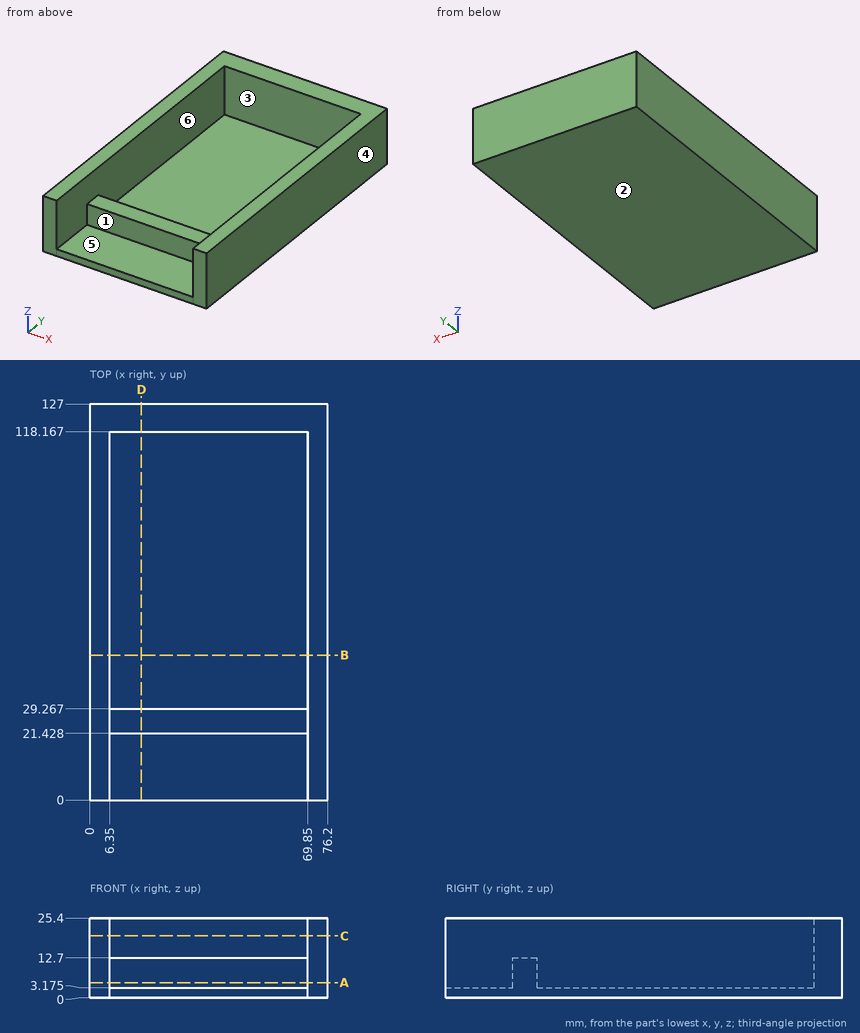
Could you check a few things on this drawing? It's one solid part, dimensions in mm from its lowest x, y, z. A direction names the side the tool comes from. Round coordinates to 2 decimals unless told otherwise and drop trailing zeros. Write each loop counter-clockwise with the first axis right and the second up, starting at its lowest first coordinate (ties: lowest second). Pieces come first, ordered by that corner, then holes.
Q1. If we section it at C-C on z = 19.75: Write out the boundary of the cut face in (x, y), plus the area to 3 significant figures.
Q2. Which directions (+Z, -Z, +X, -X, +Y, -Y) give clear straight access to the entire face, cutting with the end or side of a thin tool? Please do the marked faces 4, 5 and 6.
Q3. If we section it at A-A on z = 4.75: Write out the boundary of the cut face in (x, y).
Q4. Will these pins go through, and if not, where does the flat tip stop? P1, Ø6.5, axis at x = 34, y = 12.5, coming from the +Z side (3 decimals); P2, Ø2, axis at y = 103, z = 11, coming from the -X side; P3, Ø8, axis at x = 59, z = 13, coming from the -Y side; P4, Ø8.5, axis at x = 31, y = 26.5, coming from the +Z side.
Q5. If we mould it in two halves opening along Y, with no side actions, what happens to the marked faces 1, 2 and 3? For each: +Y half, -Y half, draft (parallel to the pull), parting line (faces both ways), or undercut.
Q6. If we section it at B-B on y = 46.5: Write out the boundary of the cut face in (x, z) (3 decimals), plus the area to 3 significant figures.
Q7. Please list where these lines run through material, in increasing order: probe 1 along X at (y, z) = (13, 20); probe 2 along Y at (x, z) = (33.5, 10.5); probe 3 along Y at (x, z) = (64, 20.75).
Q8. If we section it at D-D on x = 16.5: Write out the boundary of the cut face in (y, z) (3 decimals).
Answer below:
1. outline: (0, 0) - (6.35, 0) - (6.35, 118.17) - (69.85, 118.17) - (69.85, 0) - (76.2, 0) - (76.2, 127) - (0, 127) - close
1. area: 2,170 mm2
2. face 4: +Z, -Z, +X, +Y, -Y
2. face 5: +Z, -Y
2. face 6: +Z
3. outline: (0, 0) - (6.35, 0) - (6.35, 21.43) - (69.85, 21.43) - (69.85, 0) - (76.2, 0) - (76.2, 127) - (0, 127) - close; hole (6.35, 29.27) - (69.85, 29.27) - (69.85, 118.17) - (6.35, 118.17) - close
4. P1: stops at z = 3.175
4. P2: stops at x = 0
4. P3: stops at y = 21.43
4. P4: stops at z = 12.7
5. face 1: -Y half
5. face 2: draft
5. face 3: undercut
6. outline: (0, 0) - (76.2, 0) - (76.2, 25.4) - (69.85, 25.4) - (69.85, 3.175) - (6.35, 3.175) - (6.35, 25.4) - (0, 25.4) - close
6. area: 524 mm2
7. probe 1: x = 0 to 6.35, 69.85 to 76.2
7. probe 2: y = 21.43 to 29.27, 118.17 to 127
7. probe 3: y = 118.17 to 127
8. outline: (0, 0) - (127, 0) - (127, 25.4) - (118.167, 25.4) - (118.167, 3.175) - (29.267, 3.175) - (29.267, 12.7) - (21.428, 12.7) - (21.428, 3.175) - (0, 3.175) - close
